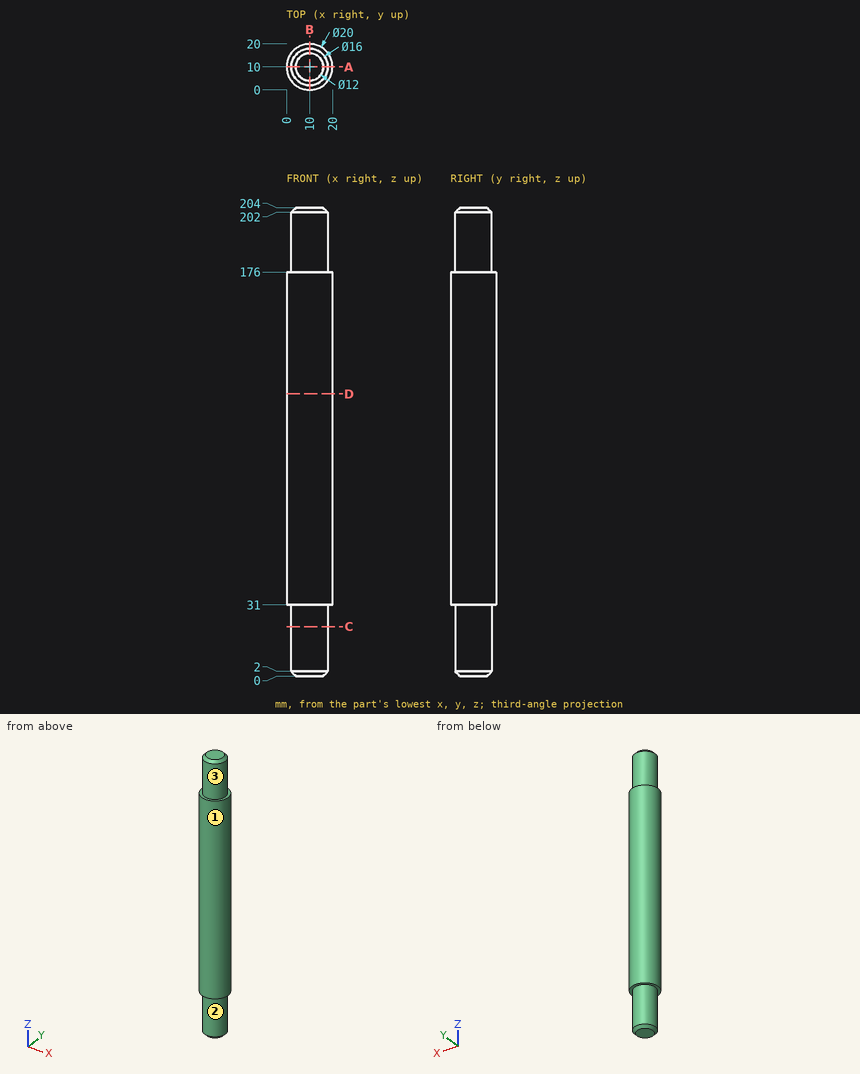
Study the drawing (mm; zero at the part's minimum x, y, z) and answer. A direction names the side the tool comes from. Round coordinates to 2 decimals unless told otherwise and drop trailing zeros. Write each loop counter-clockwise with the first axis right and the second up, starting at its lowest first coordinate (ties: lowest second). Pieces come first, ordered by that corner, then holes.
1) A cutting plane is placed at C-C (z = 21.5). Give the vertices of the cut face in (x, y), plus the area to 3 significant figures.
2) Given pin 1 Ø3 at (x, z) = (7, 128) entering from -Y; pin 2 Ø1.5 at (x, z) = (3.5, 176) entering from +Y; pin 3 Ø12 at (x, z) = (8, 148.5) entering from +Y; pin 4 Ø4 at (y, z) = (12.5, 170) entering from -X, each flat-ended and moving along its own axis, determine where each tip first touches the part or whether it passes through.
3) A cutting plane is placed at A-A (y = 10). Give the vertices of the cut face in (x, z), plus the area to 3 significant figures.
4) Straight lines are drawn through the part: line 1 (X direction, y = 2, z = 124); line 2 (X direction, y = 9.5, z = 89.5); line 3 (Z direction, x = 14.5, y = 3.25). For each, find the intervals that lie inside material, in ascending order.
5) A cutting plane is placed at D-D (z = 123). Give the vertices of the cut face in (x, y), plus the area to 3 significant figures.
6) A tool of negligible diameter and unlimited length cuts with its end or side. For the marked faces 1, 2 and 3, from which of +Z, -Z, +X, -X, +Y, -Y can it reach the whole face along a straight path? Write none if from no direction.
Completed:
1. outline: circle Ø16 at (10, 10)
1. area: 201 mm2
2. pin 1: stops at y = 0.11
2. pin 2: stops at y = 18.18
2. pin 3: stops at y = 20
2. pin 4: stops at x = 0.01
3. outline: (0, 31) - (2, 31) - (2, 2) - (4, 0) - (16, 0) - (18, 2) - (18, 31) - (20, 31) - (20, 176) - (18, 176) - (18, 202) - (16, 204) - (4, 204) - (2, 202) - (2, 176) - (0, 176) - close
3. area: 3,840 mm2
4. line 1: x = 4 to 16
4. line 2: x = 0.01 to 19.99
4. line 3: z = 31 to 176
5. outline: circle Ø20 at (10, 10)
5. area: 314 mm2
6. face 1: +Z, -Z
6. face 2: -Z
6. face 3: +Z
